Part model, mm, in its own coordinate system. A direction names the side the tool comes from. Give positions to 0.01 mm unless a question says otherwise; leave off trailing zeros. Order: outer loops, then holes, each group sorted by start corner. A loop starts at its lowest first (then second) coordinate and runs counter-clockwise, first axis right, second up.
from build123d import *

# Parameters (mm, degrees)
BASES_W            = 20.4
BASES_H            = 41
BASE_DEPTH         = 10.25
BASE_F_R           = 2
CUT_EXTRUDE3_DEPTH = 21.5


with BuildPart() as part:
    # BaseS → BASE (new body, symmetric)
    with BuildSketch(Plane(origin=(0, 0, 0), x_dir=(1, 0, 0), z_dir=(0, 1, 0))):
        Rectangle(BASES_W, BASES_H)
    extrude(amount=BASE_DEPTH, both=True)

    # BASE F
    base_f_edges = [part.edges().sort_by_distance(p)[0] for p in [
        (10.2, 0, 20.5),
        (-10.2, 0, 20.5),
        (-10.2, 0, -20.5),
        (10.2, 0, -20.5),
    ]]
    fillet(base_f_edges, radius=BASE_F_R)

    # PocketS → Cut-Extrude3 (cut, through all)
    with BuildSketch(Plane(origin=(0, 10.25, 0), x_dir=(1, 0, 0), z_dir=(0, 1, 0))):
        with BuildLine():
            Line((8.2, 19.7), (-8.2, 19.7))
            ThreePointArc((-8.2, 19.7), (-9.048528137, 19.348528137), (-9.4, 18.5))
            Line((-9.4, 18.5), (-9.4, -18.5))
            ThreePointArc((-9.4, -18.5), (-9.048528137, -19.348528137), (-8.2, -19.7))
            Line((-8.2, -19.7), (8.2, -19.7))
            ThreePointArc((8.2, -19.7), (9.048528137, -19.348528137), (9.4, -18.5))
            Line((9.4, -18.5), (9.4, 18.5))
            ThreePointArc((9.4, 18.5), (9.048528137, 19.348528137), (8.2, 19.7))
        make_face()
    extrude(amount=-CUT_EXTRUDE3_DEPTH, mode=Mode.SUBTRACT)


solid = part.part
Item 1: Which spindle directions (+Z, -Z, +X, -X, +Y, -Y) get a long thin tool onto all of the face, cutting with end or side? Do faces 1 (the face through (-9.63, -0.14, -19.9)), 2 (the face through (0, 0, -19.7)). Say none if no direction does.
Item 2: Band-saw the part on A-A on z = 0. List the corners of the cut face in (x, y), plus the area to 3 significant figures.
Item 3: Band-saw the part on C-C on y = -6.75. List the corners of the cut face in (x, z), plus the area to 3 significant figures.
Item 4: Pull direction Z, two halves, no side cores. Call faces 3 (the face through (9.4, 0, 0)), 4 (the face through (-9.4, 0, 0)), 5 (the face through (-9.63, 0.14, 19.9)), 6 (the face through (10, 10.25, -6)): released by +Z, released by -Z, zero draft, split by the parting line, or undercut.
Item 5: Band-saw the part on B-B on x = 0.5. List the corners of the cut face in (y, z), plus the area to 3 significant figures.
Item 6: Drill centre lines: probe 1 along Z at (x, y) = (2, -3); probe 2 along X at (y, z) = (3.25, -12); probe 3 along X at (y, z) = (5.5, -19). Where is each one in solid material? Low to high.
Working result:
1. face 1: -Z, -X, +Y, -Y
1. face 2: +Y, -Y
2. outline: (-10.2, -10.25) - (-9.4, -10.25) - (-9.4, 10.25) - (-10.2, 10.25) - close; (9.4, -10.25) - (10.2, -10.25) - (10.2, 10.25) - (9.4, 10.25) - close
2. area: 32.8 mm2
3. outline: (-10.2, -18.5) arc R2 ccw to (-8.2, -20.5) - (8.2, -20.5) arc R2 ccw to (10.2, -18.5) - (10.2, 18.5) arc R2 ccw to (8.2, 20.5) - (-8.2, 20.5) arc R2 ccw to (-10.2, 18.5) - close; hole (-9.4, -18.5) arc R1.2 ccw to (-8.2, -19.7) - (8.2, -19.7) arc R1.2 ccw to (9.4, -18.5) - (9.4, 18.5) arc R1.2 ccw to (8.2, 19.7) - (-8.2, 19.7) arc R1.2 ccw to (-9.4, 18.5) - close
3. area: 93.5 mm2
4. face 3: undercut
4. face 4: undercut
4. face 5: released by +Z
4. face 6: zero draft
5. outline: (-10.25, -20.5) - (10.25, -20.5) - (10.25, -19.7) - (-10.25, -19.7) - close; (-10.25, 19.7) - (10.25, 19.7) - (10.25, 20.5) - (-10.25, 20.5) - close
5. area: 32.8 mm2
6. probe 1: z = -20.5 to -19.7, 19.7 to 20.5
6. probe 2: x = -10.2 to -9.4, 9.4 to 10.2
6. probe 3: x = -10.14 to -9.29, 9.29 to 10.14
